from build123d import *

# Parameters (mm, degrees)
SKETCH1_R           = 22
BOSS_EXTRUDE1_DEPTH = 44
BOSS_EXTRUDE2_DEPTH = 13
HOLE1_D             = 22


with BuildPart() as part:
    # Sketch1 → Boss-Extrude1 (new body)
    with BuildSketch(Plane(origin=(0, 0, 0), x_dir=(1, 0, 0), z_dir=(0, 1, 0))):
        with Locations(Location((0, 0, 0), (0, 0, 270))):
            Circle(SKETCH1_R)
    extrude(amount=BOSS_EXTRUDE1_DEPTH)

    # Sketch2 → Boss-Extrude2 (add)
    with BuildSketch(Plane(origin=(0, 44, 0), x_dir=(1, 0, 0), z_dir=(0, 1, 0))):
        with BuildLine():
            Line((-12.334780679, 42.105263158), (-23.720732075, 7.894736842))
            ThreePointArc((-23.720732075, 7.894736842), (-25, 0), (-23.720732075, -7.894736842))
            Line((-23.720732075, -7.894736842), (-12.334780679, -42.105263158))
            ThreePointArc((-12.334780679, -42.105263158), (0, -51), (12.334780679, -42.105263158))
            Line((12.334780679, -42.105263158), (23.720732075, -7.894736842))
            ThreePointArc((23.720732075, -7.894736842), (25, 0), (23.720732075, 7.894736842))
            Line((23.720732075, 7.894736842), (12.334780679, 42.105263158))
            ThreePointArc((12.334780679, 42.105263158), (0, 51), (-12.334780679, 42.105263158))
        make_face()
    extrude(amount=BOSS_EXTRUDE2_DEPTH)

    # Hole1 (through all)
    with Locations(Plane(origin=(0, 57, 0), x_dir=(1, 0, 0), z_dir=(0, 1, 0))):
        with Locations((0, 0)):
            Hole(HOLE1_D / 2)

    # Sketch5 → Cut-Revolve1 (revolve, cut)
    with BuildSketch(Plane(origin=(0, 0, 0), x_dir=(0, 0, -1), z_dir=(1, 0, 0)), mode=Mode.PRIVATE) as cut_revolve1_sk:
        Polygon((0, 0), (0, 6.350852961), (-11, 6.350852961), (-22, 0), align=None)
    revolve(cut_revolve1_sk.sketch.rotate(Axis((0, 0, 0), (0, 1, 0)), 180), axis=Axis((0, 0, 0), (0, 1, 0)), mode=Mode.SUBTRACT)


solid = part.part
Design review of the part built by this model. Coordinates are the model's own, in mm. A direction names the side the tool comes from. Give positions to 0.01 mm unless a question says otherwise; leave off trailing zeros. Loops run counter-clockwise (first coordinate to the right, second up) from the corner with the lowest first, then second, coordinate; pieces in that order, holes last. Notation, with made-up numbers: (19, -13.5) -> (57, -13.5) arc R32 ccw to (57, 17.5) -> close; hole circle Ø8 at (28.25, 25.5). An arc over 180 degrees is marked (long way). One line per question, with ' | ' between items. Start each with the question number.
(1) We need section B-B (z = 0). State the section outline as (x, y) points, and give its area (3 significant figures).
(2) Insertion check: P1, Ø10, axis at x = -13, y = 15, coming from the +Z side; P2, Ø3, axis at x = -18.5, y = 9, coming from the +Z side; P3, Ø15, axis at x = 6.5, z = -9.5, coming from the -Y side. Each pin has a flat end and moves straight along its axis. Give the tip position at first contact, or say it passes through.
(3) For line 1 (Y direction, x = -11.5, z = 25.5); line 2 (Z direction, x = 3.5, y = 11); line 3 (Z direction, x = 9.5, y = 25), list the stretches that pass through material, from the lowest coordinate up.
(4) Draft analysis for pull direction Z (two halves, no side actions). For faces 1 (the face through (-10.161, 31.321, 4.213)), 2 (the face through (5, 44, 22)), 3 (the face through (10.369, 5.954, -5.393)), 4 (the face through (18.107, 50.409, -24.761)), state which applies: +Z half, -Z half, draft (parallel to the pull), parting line (faces both ways), or undercut.
(5) We need section A-A (x = 0). State the section outline as (y, z) points.
(6) For faces 5 (the face through (-21.477, 21.692, -4.769)), 6 (the face through (-11.5, 57, -0.7)), list the 3-axis set-ups (+Z, -Z, +X, -X, +Y, -Y) from which the entire face can be reached by the end or side of a thin tool; tool diameter is ignored.
(7) We need section D-D (y = 25.5). State the section outline as (x, z) points.
(8) We need section C-C (y = 50.5). State the section outline as (x, z) points, and give its area (3 significant figures).
The answers:
1) outline: (-25, 44) -> (-22, 44) -> (-22, 0) -> (-11, 6.35) -> (-11, 57) -> (-25, 57) -> close; (11, 6.35) -> (22, 0) -> (22, 44) -> (25, 44) -> (25, 57) -> (11, 57) -> close | area: 1,260 mm^2
2) P1: stops at z = 20.49 | P2: stops at z = 13.96 | P3: stops at y = 1.73
3) line 1: y = 44 to 57 | line 2: z = -21.72 to -10.43, 10.43 to 21.72 | line 3: z = -19.84 to -5.55, 5.55 to 19.84
4) face 1: undercut | face 2: draft | face 3: undercut | face 4: -Z half
5) outline: (0, -22) -> (44, -22) -> (44, -51) -> (57, -51) -> (57, -11) -> (6.35, -11) -> close; (0, 22) -> (6.35, 11) -> (57, 11) -> (57, 51) -> (44, 51) -> (44, 22) -> close
6) face 5: -Y | face 6: +Z, -Z, +X, -X, +Y
7) outline: circle Ø44 at (0, 0); hole circle Ø22 at (0, 0)
8) outline: (-23.72, -7.89) -> (-12.33, -42.11) arc R13 ccw to (12.33, -42.11) -> (23.72, -7.89) arc R25 ccw to (23.72, 7.89) -> (12.33, 42.11) arc R13 ccw to (-12.33, 42.11) -> (-23.72, 7.89) arc R25 ccw to start; hole circle Ø22 at (0, 0) | area: 3,180 mm^2
